```python
from build123d import *

# Parameters (mm, degrees)
BOSS_EXTRUDE4_DEPTH = 10
SKETCH6_R           = 1.6
CUT_EXTRUDE2_DEPTH  = 47.135107158
FILLET4_R           = 5
SKETCH7_W           = 4
SKETCH7_H           = 12
BOSS_EXTRUDE5_DEPTH = 15
FILLET5_START       = -10.0000001
FILLET5_DEPTH       = 10.0000001
FILLET5_START_2     = -22
FILLET5_2_DEPTH     = 44
FILLET6_R           = 2


with BuildPart() as part:
    # Sketch5 → Boss-Extrude4 (new body)
    with BuildSketch(Plane(origin=(0, 0, 0), x_dir=(1, 0, 0), z_dir=(0, 1, 0))):
        with BuildLine():
            ThreePointArc((17.3, 0), (-10.314795199, -13.888664443), (-5, 16.561702811))
            Line((-5, 16.561702811), (-5, 20.704830354))
            ThreePointArc((-5, 20.704830354), (-13.17554553, -16.736038958), (21.3, 0))
            ThreePointArc((21.3, 0), (16.736038958, 13.17554553), (5, 20.704830354))
            Line((5, 20.704830354), (5, 16.561702811))
            ThreePointArc((5, 16.561702811), (13.888664443, 10.314795199), (17.3, 0))
        make_face()
        with BuildLine():
            ThreePointArc((-5, 20.704830354), (-3.013586771, 21.085736761), (-1, 21.276512872))
            Line((-1, 21.276512872), (-1, 36.561702811))
            Line((-1, 36.561702811), (-5, 36.561702811))
            Line((-5, 36.561702811), (-5, 20.704830354))
        make_face()
        with BuildLine():
            ThreePointArc((-5, 16.561702811), (-3.020894222, 17.034206706), (-1, 17.271074084))
            Line((-1, 17.271074084), (-1, 21.276512872))
            ThreePointArc((-1, 21.276512872), (-3.013586771, 21.085736761), (-5, 20.704830354))
            Line((-5, 20.704830354), (-5, 16.561702811))
        make_face()
        with BuildLine():
            Line((1, 21.276512872), (1, 17.271074084))
            ThreePointArc((1, 17.271074084), (3.020894222, 17.034206706), (5, 16.561702811))
            Line((5, 16.561702811), (5, 20.704830354))
            ThreePointArc((5, 20.704830354), (3.013586771, 21.085736761), (1, 21.276512872))
        make_face()
        with BuildLine():
            Line((1, 36.561702811), (1, 21.276512872))
            ThreePointArc((1, 21.276512872), (3.013586771, 21.085736761), (5, 20.704830354))
            Line((5, 20.704830354), (5, 36.561702811))
            Line((5, 36.561702811), (1, 36.561702811))
        make_face()
    extrude(amount=BOSS_EXTRUDE4_DEPTH)

    # Sketch6 → Cut-Extrude2 (cut, through all)
    with BuildSketch(Plane(origin=(5, 0, 0), x_dir=(0, 0, -1), z_dir=(1, 0, 0))):
        with Locations((28.561702811, 5)):
            Circle(SKETCH6_R)
    extrude(amount=-CUT_EXTRUDE2_DEPTH, mode=Mode.SUBTRACT)

    # Fillet4
    fillet4_edges = [part.edges().sort_by_distance(p)[0] for p in [
        (5, 5, -20.704830354),
        (-5, 5, -20.704830354),
    ]]
    fillet(fillet4_edges, radius=FILLET4_R)

    # Sketch7 → Boss-Extrude5 (add)
    with BuildSketch(Plane.XZ):
        with Locations((-3, -30.561702811)):
            Rectangle(SKETCH7_W, SKETCH7_H)
        with Locations((3, -30.561702811)):
            Rectangle(SKETCH7_W, SKETCH7_H)
    extrude(amount=BOSS_EXTRUDE5_DEPTH)

    # Fillet5: read off the stored shape, not the designer's step
    # Fillet5 outline → Fillet5 (add)
    with BuildSketch(Plane(origin=(0, 0, 0), x_dir=(1, 0, 0), z_dir=(0, 1, 0)).offset(FILLET5_START)):
        with BuildLine():
            Line((-1, 17.271074084), (-1, 24.561702811))
            Line((-1, 24.561702811), (-5, 24.561702811))
            Line((-5, 24.561702811), (-5, 24.324678826))
            ThreePointArc((-5, 24.324678826), (-5.846344777, 21.541308874), (-8.098859316, 19.700215171))
            ThreePointArc((-8.098859316, 19.700215171), (0, -21.3), (8.098859316, 19.700215171))
            ThreePointArc((8.098859316, 19.700215171), (5.846344777, 21.541308874), (5, 24.324678826))
            Line((5, 24.324678826), (5, 24.561702811))
            Line((5, 24.561702811), (1, 24.561702811))
            Line((1, 24.561702811), (1, 17.271074084))
            ThreePointArc((1, 17.271074084), (0, -17.3), (-1, 17.271074084))
        make_face()
    extrude(amount=FILLET5_DEPTH)

    # Fillet5 2 outline → Fillet5 2 (cut)
    with BuildSketch(Plane.YZ.offset(FILLET5_START_2)):
        with BuildLine():
            ThreePointArc((-10, -24.561702811), (-2.928932188, -21.632770623), (0, -14.561702811))
            Line((0, -14.561702811), (0, 23))
            Line((0, 23), (-10.0000001, 23))
            Line((-10.0000001, 23), (-10, -24.561702811))
        make_face()
    extrude(amount=FILLET5_2_DEPTH, mode=Mode.SUBTRACT)

    # Fillet6
    fillet6_edges = [part.edges().sort_by_distance(p)[0] for p in [
        (5, -2.5, -36.561702811),
        (1, -2.5, -36.561702811),
        (-1, -2.5, -36.561702811),
        (-5, -2.5, -36.561702811),
    ]]
    fillet(fillet6_edges, radius=FILLET6_R - 0.0001)  # a hair under: the kernel refuses the full size


solid = part.part
```
Source: CAD feature listing. Evaluate the final solid. Frame: model axes, mm. A direction names the side the tool comes from. Coordinates: 2 decimals unless noted, no trailing zeros. Write each loop counter-clockwise with the first axis right and the second up, starting at its lowest first coordinate (ties: lowest second). Pieces come first, ordered by that corner, then holes. Notation, with made-up numbers: (-17.5, 19.25) -> (29.5, 19.25) arc R25 ccw to (29.5, 58.25) -> close; hole circle Ø10 at (-32, -20). An arc over 180 degrees is marked (long way). Return JSON: item names as keys, results as strings. Group by question number.
1) Mould query, pull axis Z, two halves, no side actions, for faces 1 (the face through (-4.4, -2.68, -35.99)), 2 (the face through (-2.97, 3.58, -29.3)), 3 (the face through (3, -12, -24.562)). Classes: +Z half, -Z half, draft (parallel to the pull), parting line (faces both ways), or undercut.
2) Contact query for flat-ended pins moving along their axis: P1, Ø2, axis at x = -7.5, z = -22.5, coming from the -Y side; P2, Ø5, axis at y = 1.5, z = -23, coming from the -X side; P3, Ø5, axis at y = 5, z = -28.56, coming from the -X side; P4, Ø12, axis at x = 7.5, y = -12, coming from the +Z side. Output: stop coordinate, or through.
3) Section query B-B, the plane z = 1. Return loops of the section in (x, y).
4) Set-up query: faces 4 (the face through (-5, -3, -30)), 5 (the face through (5, -3, -29)), 6 (the face through (3, -15, -30)), 7 (the face through (0, 0, 18)), 8 (the face through (1, 0, -28)). Return all of +Z, -Z, +X, -X, +Y, -Y with unobstructed straight access to the full face (end or side cutting, diameter ignored); none if empty.
5) Section query D-D, the plane x = 11. Return loops of the section in (y, z), plus the area to 3 significant figures.
6) Ray query, line 1 along X through (y, z) = (-3, -25); line 2 along Z through (x, y) = (-2.5, 4); line 3 along Y through (x, z) = (-6.5, 18). Return the intervals inside material, ascending.
7) Section query C-C, the plane y = 5. State how many separate pieces and enclosed holes the cut face has, plus the area to 3 significant figures.
From the geometry:
{
 "1": {"face 1": "-Z half", "face 2": "undercut", "face 3": "+Z half"},
 "2": {"P1": "through", "P2": "x = -6.78", "P3": "x = -5", "P4": "z = -23.94"},
 "3": {"outline": "(-21.28, 0) -> (-17.27, 0) -> (-17.27, 10) -> (-21.28, 10) -> close; (17.27, 0) -> (21.28, 0) -> (21.28, 10) -> (17.27, 10) -> close"},
 "4": {"face 4": "-Z, -X, +Y, -Y", "face 5": "-Z, +X, +Y, -Y", "face 6": "+Z, -Z, +X, -X, -Y", "face 7": "+Z, +X, -X, -Y", "face 8": "-Z, +Y, -Y"},
 "5": {"outline": "(-0.7, -18.24) -> (10, -18.24) -> (10, -13.35) -> (0, -13.35) -> (0, -14.56) arc R10 cw to start; (0, 13.35) -> (10, 13.35) -> (10, 18.24) -> (0, 18.24) -> close", "area": "98.6 mm²"},
 "6": {"line 1": "-5 to -1, 1 to 5", "line 2": "-36.5 to -29.81, -27.31 to -17.12, 17.12 to 21.15", "line 3": "0 to 10"},
 "7": {"separate pieces": "3", "enclosed holes": "0", "area": "577 mm²"}
}
